from build123d import *

# Parameters (mm, degrees)
BOSS_EXTRUDE1_DEPTH = 5
SCALE2_SCALE        = 0.265
SKETCH6_W           = 6.3
SKETCH6_H           = 17.1
BOSS_EXTRUDE2_DEPTH = 1.325
SKETCH5_W           = 11.5
SKETCH5_H           = 9
SKETCH5_R           = 1.468522593
CUT_EXTRUDE1_DEPTH  = 1.325
SKETCH8_R           = 1.5
BOSS_EXTRUDE5_DEPTH = 15.9


with BuildPart() as part:
    # Sketch1 → Boss-Extrude1 (new body)
    with BuildSketch(Plane(origin=(0, 0, 0), x_dir=(1, 0, 0), z_dir=(0, 1, 0))):
        with BuildLine():
            Line((-247.677130459, 9.093460821), (0, 9.093460821))
            Line((0, 9.093460821), (1.981474539, 9.093460821))
            Line((1.981474539, 9.093460821), (3.962949079, 9.093460821))
            Line((3.962949079, 9.093460821), (251.640079537, 9.093460821))
            ThreePointArc((251.640079537, 9.093460821), (261.186021083, 13.047519275), (265.140079537, 22.593460821))
            Line((265.140079537, 22.593460821), (265.140079537, 87.593460821))
            Line((265.140079537, 87.593460821), (265.140079537, 152.207743366))
            Line((265.140079537, 152.207743366), (265.140079537, 196.397667024))
            ThreePointArc((265.140079537, 196.397667024), (261.186021083, 205.94360857), (251.640079537, 209.897667024))
            Line((251.640079537, 209.897667024), (171.71214435, 209.897667024))
            ThreePointArc((171.71214435, 209.897667024), (167.885310027, 210.658871699), (164.641076538, 212.826599212))
            Line((164.641076538, 212.826599212), (154.53187981, 222.935795941))
            ThreePointArc((154.53187981, 222.935795941), (152.364152296, 226.180029429), (151.602947621, 230.006863753))
            Line((151.602947621, 230.006863753), (151.602947621, 238.96110688))
            ThreePointArc((151.602947621, 238.96110688), (147.209549339, 249.567708598), (136.602947621, 253.96110688))
            Line((136.602947621, 253.96110688), (3.962949079, 253.96110688))
            Line((3.962949079, 253.96110688), (0, 253.96110688))
            Line((0, 253.96110688), (-132.639998543, 253.96110688))
            ThreePointArc((-132.639998543, 253.96110688), (-143.246600261, 249.567708598), (-147.639998543, 238.96110688))
            Line((-147.639998543, 238.96110688), (-147.639998543, 230.006863753))
            ThreePointArc((-147.639998543, 230.006863753), (-148.401203218, 226.180029429), (-150.568930731, 222.935795941))
            Line((-150.568930731, 222.935795941), (-160.67812746, 212.826599212))
            ThreePointArc((-160.67812746, 212.826599212), (-163.922360948, 210.658871699), (-167.749195272, 209.897667024))
            Line((-167.749195272, 209.897667024), (-247.677130459, 209.897667024))
            ThreePointArc((-247.677130459, 209.897667024), (-257.223072005, 205.94360857), (-261.177130459, 196.397667024))
            Line((-261.177130459, 196.397667024), (-261.177130459, 152.207743366))
            Line((-261.177130459, 152.207743366), (-261.177130459, 87.593460821))
            Line((-261.177130459, 87.593460821), (-261.177130459, 22.593460821))
            ThreePointArc((-261.177130459, 22.593460821), (-257.223072005, 13.047519275), (-247.677130459, 9.093460821))
        make_face()
    extrude(amount=BOSS_EXTRUDE1_DEPTH)


with BuildPart() as part_1:
    # Scale2: scaled about (0, 0, 0)
    add(part.part.scale(SCALE2_SCALE))

    # Sketch6 → Boss-Extrude2 (add)
    with BuildSketch(Plane(origin=(0, 1.325, 0), x_dir=(1, 0, 0), z_dir=(0, 1, 0))):
        with Locations((-72.361939572, 31.762267118)):
            Rectangle(SKETCH6_W, SKETCH6_H)
        with Locations((73.412121077, 31.762267118)):
            Rectangle(SKETCH6_W, SKETCH6_H)
    extrude(amount=-BOSS_EXTRUDE2_DEPTH)

    # Sketch5 → Cut-Extrude1 (cut)
    with BuildSketch(Plane(origin=(0, 1.325, 0), x_dir=(1, 0, 0), z_dir=(0, 1, 0))):
        Polygon((-67.511939572, 27.772881761), (-67.511939572, 20.272881761), (-55.711939572, 20.272881761), (-55.711939572, 4.922881761), (-40.711939572, 4.922881761), (-40.711939572, 20.272881761), (-27.461939572, 20.272881761), (-27.461939572, 9.799693323), (28.538060428, 9.799693323), (28.538060428, 20.272881761), (41.762121077, 20.272881761), (41.762121077, 4.922881761), (56.762121077, 4.922881761), (56.762121077, 20.272881761), (68.562121077, 20.272881761), (68.562121077, 35.272881761), (56.762121077, 35.272881761), (56.762121077, 50.622881761), (41.762121077, 50.622881761), (41.762121077, 35.272881761), (28.538060428, 35.272881761), (28.538060428, 44.799693323), (-27.461939572, 44.799693323), (-27.461939572, 35.272881761), (-40.711939572, 35.272881761), (-40.711939572, 50.622881761), (-55.711939572, 50.622881761), (-55.711939572, 35.272881761), (-67.511939572, 35.272881761), align=None)
        with Locations((-29.874599614, 61.299693323)):
            Rectangle(SKETCH5_W, SKETCH5_H)
        with Locations((-35.711939572, 42.772881761)):
            Circle(SKETCH5_R)
        with Locations((-60.711939572, 42.772881761)):
            Circle(SKETCH5_R)
        with Locations((-60.711939572, 12.772881761)):
            Circle(SKETCH5_R)
        with Locations((-35.711939572, 12.772881761)):
            Circle(SKETCH5_R)
        with Locations((36.762121077, 12.772881761)):
            Circle(SKETCH5_R)
        with Locations((61.762121077, 12.772881761)):
            Circle(SKETCH5_R)
        with Locations((36.762121077, 42.772881761)):
            Circle(SKETCH5_R)
        with Locations((61.762121077, 42.772881761)):
            Circle(SKETCH5_R)
    extrude(amount=-CUT_EXTRUDE1_DEPTH, mode=Mode.SUBTRACT)

    # Sketch8 → Boss-Extrude5 (add)
    with BuildSketch(Plane(origin=(0, 1.325, 0), x_dir=(1, 0, 0), z_dir=(0, 1, 0))):
        with Locations((-72.861939572, 36.019267118)):
            Circle(SKETCH8_R)
        with Locations((-72.861939572, 27.505267118)):
            Circle(SKETCH8_R)
        with Locations((73.912121077, 36.019267118)):
            Circle(SKETCH8_R)
        with Locations((73.912121077, 27.505267118)):
            Circle(SKETCH8_R)
    extrude(amount=BOSS_EXTRUDE5_DEPTH)


solid = part_1.part
CAD build for the part. Positions are in the model's coordinates, mm. A direction names the side the tool comes from. Give positions to 0.01 mm unless a question says otherwise; leave off trailing zeros. Order: outer loops, then holes, each group sorted by start corner. A loop starts at its lowest first (then second) coordinate and runs counter-clockwise, first axis right, second up. Notation, with made-up numbers: (25, 67.25) -> (78, 67.25) arc R10 cw to (78, 72.25) -> close; hole circle Ø9 at (10.5, 32.5). An arc over 180 degrees is marked (long way). Return JSON: item names as keys, results as strings.
Q1. Mould opens along Z. For faces 3 (the face through (-34.355, 0.672, -12.21)), 4 (the face through (69.24, 0.65, -54.55)), 5 (the face through (-73, 17.225, -28)) say: pulls with the +Z half, pulls with the -Z half, needs draft (parallel to the pull), parting line crosses it, or undercut.
Working result:
{"face 3": "undercut", "face 4": "pulls with the -Z half", "face 5": "needs draft"}
Q2. Saw through at B-B (x = -53). Write the cut outline in (y, z) (3 decimals), then the cut area to 3 significant figures.
Working result:
{"outline": "(0, -55.623) -> (1.325, -55.623) -> (1.325, -50.623) -> (0, -50.623) -> close; (0, -4.923) -> (1.325, -4.923) -> (1.325, -2.41) -> (0, -2.41) -> close", "area": "9.95 mm²"}
Q3. Saw through at C-C (z = -18.5). Write the cut outline in (x, y) (3 decimals), then the cut area to 3 significant figures.
Working result:
{"outline": "(-69.212, 0) -> (-55.712, 0) -> (-55.712, 1.325) -> (-69.212, 1.325) -> close; (-40.712, 0) -> (-27.462, 0) -> (-27.462, 1.325) -> (-40.712, 1.325) -> close; (28.538, 0) -> (41.762, 0) -> (41.762, 1.325) -> (28.538, 1.325) -> close; (56.762, 0) -> (70.262, 0) -> (70.262, 1.325) -> (56.762, 1.325) -> close", "area": "70.9 mm²"}
Q4. Which spindle directions (+Z, -Z, +X, -X, +Y, -Y) get a long thin tool onto all of the face, cutting with end or side? Do faces 1 (the face through (-36.03, 0.67, -41.34)), 2 (the face through (72.72, 9.16, -35.11)). Say none if no direction does.
Working result:
{"face 1": "+Y, -Y", "face 2": "+Y"}
Q5. Saw through at D-D (x = 22.5). Write the cut outline in (y, z) (3 decimals), then the cut area to 3 significant figures.
Working result:
{"outline": "(0, -67.3) -> (1.325, -67.3) -> (1.325, -44.8) -> (0, -44.8) -> close; (0, -9.8) -> (1.325, -9.8) -> (1.325, -2.41) -> (0, -2.41) -> close", "area": "39.6 mm²"}
Q6. Flat gauge pins, fed straight in: pin 1 (1.5 mm diameter, centred on y = 1, z = -63.5, fed in from +X); pin 2 (0.7 mm diameter, centred on y = 1, z = -43.5, fed in from -X); pin 3 (12 mm diameter, centred on x = 21, z = -60, fed in from +Y) (3 decimals). Where does each tip first touch, or does it go through?
Working result:
{"pin 1": "x = 40.17", "pin 2": "x = -69.21", "pin 3": "y = 1.325"}
Q7. Saw through at A-A (z = -47). Write the cut outline in (x, y) (3 decimals), then the cut area to 3 significant figures.
Working result:
{"outline": "(-69.212, 0) -> (-55.712, 0) -> (-55.712, 1.325) -> (-69.212, 1.325) -> close; (-40.712, 0) -> (41.762, 0) -> (41.762, 1.325) -> (-40.712, 1.325) -> close; (56.762, 0) -> (70.262, 0) -> (70.262, 1.325) -> (56.762, 1.325) -> close", "area": "145 mm²"}
Q8. Drill centre lines: line 1 (Z direction, x = -9, y = 1); line 2 (X direction, y = 4.5, z = -28); line 3 (X direction, y = 9.75, z = -35.5). Where is each one in solid material? Low to high.
Working result:
{"line 1": "-67.3 to -44.8, -9.8 to -2.41", "line 2": "-74.28 to -71.45, 72.5 to 75.33", "line 3": "-74.27 to -71.45, 72.5 to 75.32"}
